Verification items for the finished model (mm, model axes). Face numbers are marked on the shaded views. A direction names the side the tool comes from. Coordinates: 2 decimals unless noted, no trailing zeros. Write each loop counter-clockwise with the first axis right and the second up, starting at its lowest first coordinate (ties: lowest second). Pieces come first, ordered by that corner, then holes. Notation, with made-up numbers: (55.25, 69.25) -> (62.25, 69.25) arc R19 ccw to (62.25, 88.25) -> close; hole circle Ø10 at (-27.5, 66). An arc over 180 degrees is marked (long way). Write each question's results on one line, items separated by ' | '. Start each with the question number.
from build123d import *

# Parameters (mm, degrees)
SKETCH1_R           = 2.4
BOSS_EXTRUDE1_DEPTH = 56.59882
SKETCH7_W           = 12.7
SKETCH7_H           = 12.7
BOSS_EXTRUDE3_DEPTH = 12.7
CUT_EXTRUDE2_REACH  = 228.355
SKETCH8_R           = 2.625
FILLET1_R           = 5.08


with BuildPart() as part:
    # Sketch1 → Boss-Extrude1 (new body)
    with BuildSketch(Plane.XY):
        with BuildLine():
            Line((-77.443191063, 182.115759687), (-79.348229949, 182.102566798))
            Line((-79.348229949, 182.102566798), (-80.618191063, 204.196458108))
            ThreePointArc((-80.618191063, 204.196458108), (-82.664050197, 209.135598974), (-87.603191063, 211.181458108))
            Line((-87.603191063, 211.181458108), (-87.603191063, 208.926458108))
            ThreePointArc((-87.603191063, 208.926458108), (-93.603191063, 202.926458108), (-99.603191063, 208.926458108))
            Line((-99.603191063, 208.926458108), (-99.603191063, 214.356458108))
            Line((-99.603191063, 214.356458108), (-90.238191127, 214.356458108))
            Line((-90.238191127, 214.356458108), (-87.603191063, 214.356458108))
            Line((-87.603191063, 214.356458108), (-76.173191063, 214.356458108))
            Line((-76.173191063, 214.356458108), (-53.948191063, 214.356458108))
            Line((-53.948191063, 214.356458108), (-53.948191063, 195.941458108))
            Line((-53.948191063, 195.941458108), (-57.123191063, 195.941458108))
            Line((-57.123191063, 195.941458108), (-57.123191063, 208.641458108))
            ThreePointArc((-57.123191063, 208.641458108), (-57.867139839, 210.437509332), (-59.663191063, 211.181458108))
            Line((-59.663191063, 211.181458108), (-75.706469876, 211.181458108))
            ThreePointArc((-75.706469876, 211.181458108), (-77.79329282, 210.089480898), (-78.085814114, 207.752458108))
            ThreePointArc((-78.085814114, 207.752458108), (-77.605137508, 206.003257791), (-77.443191063, 204.196458108))
            Line((-77.443191063, 204.196458108), (-77.443191063, 182.115759687))
        make_face()
        with Locations((-93.603191063, 208.926458108)):
            Circle(SKETCH1_R, mode=Mode.SUBTRACT)
    extrude(amount=BOSS_EXTRUDE1_DEPTH)

    # Sketch7 → Boss-Extrude3 (add)
    with BuildSketch(Plane(origin=(-53.948191063, 0, 0), x_dir=(0, 0, -1), z_dir=(1, 0, 0))):
        with Locations((-50.24882, 202.291458108)):
            Rectangle(SKETCH7_W, SKETCH7_H)
        with Locations((-6.35, 202.291458108)):
            Rectangle(SKETCH7_W, SKETCH7_H)
    extrude(amount=-BOSS_EXTRUDE3_DEPTH)

    # Sketch8 → Cut-Extrude2 (cut, up to next)
    with BuildSketch(Plane(origin=(-53.948191063, 0, 0), x_dir=(0, 0, -1), z_dir=(1, 0, 0)), mode=Mode.PRIVATE) as cut_extrude2_sk1:
        with Locations((-50.24882, 202.291458108)):
            Circle(SKETCH8_R)
    cut_extrude2_tool1 = extrude(cut_extrude2_sk1.sketch, amount=-CUT_EXTRUDE2_REACH, mode=Mode.PRIVATE) & part.part
    # Sketch8 → Cut-Extrude2 (cut, up to next)
    with BuildSketch(Plane(origin=(-53.948191063, 0, 0), x_dir=(0, 0, -1), z_dir=(1, 0, 0)), mode=Mode.PRIVATE) as cut_extrude2_sk2:
        with Locations((-6.35, 202.291458108)):
            Circle(SKETCH8_R)
    cut_extrude2_tool2 = extrude(cut_extrude2_sk2.sketch, amount=-CUT_EXTRUDE2_REACH, mode=Mode.PRIVATE) & part.part
    add(cut_extrude2_tool1.solids().sort_by_distance((-53.948191, 202.291458, 50.24882))[0], mode=Mode.SUBTRACT)
    add(cut_extrude2_tool2.solids().sort_by_distance((-53.948191, 202.291458, 6.35))[0], mode=Mode.SUBTRACT)

    # Fillet1
    fillet1_edges = [part.edges().sort_by_distance(p)[0] for p in [
        (-53.948191063, 214.356458108, 28.29941),
    ]]
    fillet(fillet1_edges, radius=FILLET1_R)


solid = part.part
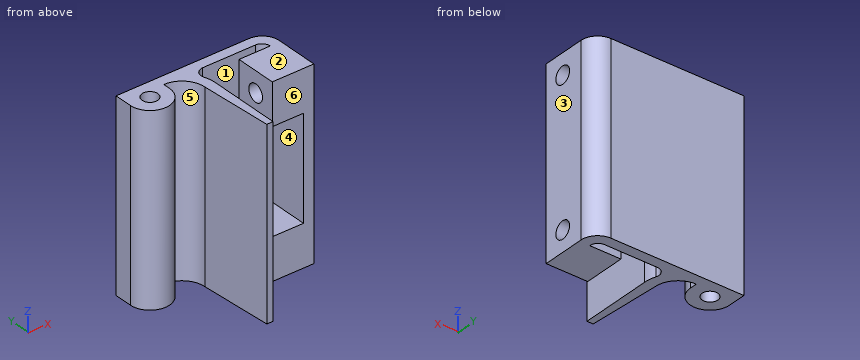
1. Material ranges on probe 1 along Y at (x, z) = (-61.5, 6.35); probe 2 along Z at (x, y) = (-63, 202.5); probe 3 along Y at (x, z) = (-60.5, 10), recorded low to high. Write a range as from..to.
2. Sectioned sample at D-D on x = -85. Record the cut outline in (y, z), plus the area to 3 significant figures.
3. Sectioned sample at A-A on z = 6.35. Record the cut outline in (x, y) (3 decimals).
4. Depth check by flat-ended pin: pin 1 Ø4.5 at (y, z) = (202.29, 50.25) entering from +X; pin 2 Ø10.5 at (x, y) = (-60, 201) entering from -Z; pin 3 Ø5 at (y, z) = (195, 23.5) entering from -X; pin 4 Ø2 at (x, z) = (-69.5, 39.5) entering from -Y. Enter the tip coordinate at first touch or a pass-through.
5. Sectioned sample at C-C on y = 194. Record the cut outline in (x, z).
6. Mould release check, pull along X, two halves, no side actions. Record for the marked faces 1, 2 and 3: +X half, -X half, draft (parallel to the pull), parting line (faces both ways), or undercut.
7. Sectioned sample at B-B on z = 35. Record the cut outline in (x, y) (3 decimals).
8. Tool access check on the marked faces 4, 5 and 6. Record the directions out of +Z, -Z, +X, -X, +Y, -Y that give a thin tool (end or side, any length) a straight path to the whole face; none if there is none.
Computed values:
1) probe 1: y = 195.94..199.67, 204.92..208.64, 211.18..214.36 | probe 2: z = 0..3.73, 8.97..12.7, 43.9..47.63, 52.87..56.6 | probe 3: y = 195.94..208.64, 211.18..214.36
2) outline: (210.68, 0) -> (214.36, 0) -> (214.36, 56.6) -> (210.68, 56.6) -> close | area: 208 mm^2
3) outline: (-99.603, 208.926) arc R6 ccw to (-87.603, 208.926) -> (-87.603, 211.181) arc R6.985 cw to (-80.618, 204.196) -> (-79.348, 182.103) -> (-77.443, 182.116) -> (-77.443, 204.196) arc R10.16 ccw to (-78.086, 207.752) arc R2.54 cw to (-75.706, 211.181) -> (-59.663, 211.181) arc R2.54 cw to (-57.123, 208.641) -> (-66.648, 208.641) -> (-66.648, 204.916) -> (-53.948, 204.916) -> (-53.948, 209.276) arc R5.08 ccw to (-59.028, 214.356) -> (-99.603, 214.356) -> close; (-66.648, 195.941) -> (-53.948, 195.941) -> (-53.948, 199.666) -> (-66.648, 199.666) -> close; hole circle Ø4.8 at (-93.603, 208.926)
4) pin 1: stops at x = -77.44 | pin 2: stops at z = 0 | pin 3: stops at x = -80.23 | pin 4: stops at y = 211.18
5) outline: (-80.03, 0) -> (-77.44, 0) -> (-77.44, 56.6) -> (-80.03, 56.6) -> close
6) face 1: undercut | face 2: draft | face 3: +X half
7) outline: (-99.603, 208.926) arc R6 ccw to (-87.603, 208.926) -> (-87.603, 211.181) arc R6.985 cw to (-80.618, 204.196) -> (-79.348, 182.103) -> (-77.443, 182.116) -> (-77.443, 204.196) arc R10.16 ccw to (-78.086, 207.752) arc R2.54 cw to (-75.706, 211.181) -> (-59.663, 211.181) arc R2.54 cw to (-57.123, 208.641) -> (-57.123, 195.941) -> (-53.948, 195.941) -> (-53.948, 209.276) arc R5.08 ccw to (-59.028, 214.356) -> (-99.603, 214.356) -> close; hole circle Ø4.8 at (-93.603, 208.926)
8) face 4: -Y | face 5: +Z, -Z, -Y | face 6: +Z, -Z, +X, -Y
